Verification items for the finished model (mm, model axes). Give positions to 0.01 mm unless a question says otherwise; leave off trailing zeros. Order: outer loops, then holes, each group sorted by start corner. A loop starts at its lowest first (then second) coordinate and runs counter-clockwise, first axis right, second up. Notation, with made-up numbers: (16.25, 51.25) - (75.25, 51.25) arc R16 cw to (75.25, 56.25) - close; hole circle Ø9 at (51, 17). An arc over 180 degrees is marked (long way). Answer as a JSON object with one key per item and string values. Group by question number.
(1) Section check A-A (z = 0). Record the boundary of the cut face in (x, y), then the cut area to 3 significant figures.
(2) Depth check by flat-ended pin: pin 1 Ø4 at (x, z) = (-1.5, 0.5) entering from +Y. Enter the tip coordinate at first touch or a pass-through.
(3) Section check C-C (y = 0.8). Record the boundary of the cut face in (x, z) (1 decimal).
(4) Thickness scan on line 1 (X direction, y = 2.6, z = -0.5); line 2 (Z direction, x = 10.5, y = 1.3); line 3 (Z direction, x = -0.25, y = 2.85). Record the ranges inside material, lowest first.
(5) Section check B-B (x = 0). Record the boundary of the cut face in (y, z), then the cut area to 3 significant figures.
(6) Section check D-D (z = 4). Record the boundary of the cut face in (x, y).
(7) Mould release check, pull along Z, two halves, no side actions. Record for faces 1 (the face through (4, 3, 0)), 2 (the face through (12, 1, 0)), 3 (the face through (0.9, 1.48, 2.86)), 4 (the face through (5.747, 1.479, 3.164)): +Z half, -Z half, draft (parallel to the pull), parting line (faces both ways), or undercut.
```python
from build123d import *

# Parameters (mm, degrees)
SKETCH_1_R      = 4.5
SKETCH_1_R_2    = 3
SKETCH_1_R_3    = 2
EXTRUDE_1_DEPTH = 3


with BuildPart() as part:
    # 草图1 → 凸台-拉伸1 (new body)
    # profile 1 of 3: a face of its own
    with BuildSketch(Plane(origin=(0, 0, 0), x_dir=(1, 0, 0), z_dir=(0, 1, 0))):
        Circle(SKETCH_1_R)
        with Locations(Location((0, 0, 0), (0, 0, 270))):
            Circle(SKETCH_1_R_2, mode=Mode.SUBTRACT)
    # profile 2 of 3: a face of its own
    with BuildSketch(Plane(origin=(0, 0, 0), x_dir=(1, 0, 0), z_dir=(0, 1, 0))):
        with BuildLine():
            ThreePointArc((10.5, -1.936491675), (8, -2e-09), (10.5, 1.936491671))
            Line((10.5, 1.936491671), (1.125000001, 4.357106264))
            ThreePointArc((1.125000001, 4.357106264), (3.557562368, 2.75567596), (4.5, 0))
            ThreePointArc((4.5, 0), (3.557562367, -2.755675961), (1.124999999, -4.357106265))
            Line((1.124999999, -4.357106265), (10.5, -1.936491675))
        make_face()
    # profile 3 of 3: a face of its own
    with BuildSketch(Plane(origin=(0, 0, 0), x_dir=(1, 0, 0), z_dir=(0, 1, 0))):
        with Locations((10, -2e-09)):
            Circle(SKETCH_1_R_3)
    extrude(amount=EXTRUDE_1_DEPTH)


solid = part.part
```
Solutions:
{
 "1": {"outline": "(-4.5, 0) - (-3, 0) - (-3, 3) - (-4.5, 3) - close; (3, 0) - (12, 0) - (12, 3) - (3, 3) - close", "area": "31.5 mm2"},
 "2": {"pin 1": "stops at y = 3"},
 "3": {"outline": "(1.1, -4.4) - (10.5, -1.9) arc R2 ccw to (10.5, 1.9) - (1.1, 4.4) arc R4.5 ccw (long way) to start; hole circle Ø6 at (0, 0)"},
 "4": {"line 1": "x = -4.47 to -2.96, 2.96 to 11.94", "line 2": "z = -1.94 to 1.94", "line 3": "z = -4.49 to -2.99, 2.99 to 4.49"},
 "5": {"outline": "(0, -4.5) - (3, -4.5) - (3, -3) - (0, -3) - close; (0, 3) - (3, 3) - (3, 4.5) - (0, 4.5) - close", "area": "9.00 mm2"},
 "6": {"outline": "(-2.06, 0) - (2.51, 0) - (2.51, 3) - (-2.06, 3) - close"},
 "7": {"face 1": "draft", "face 2": "parting line", "face 3": "undercut", "face 4": "+Z half"}
}
